Can you work these out from the model? Positions are in its coordinate system, mm. A direction names the side the tool comes from. Give positions to 0.01 mm unless a question says otherwise; leave off trailing zeros. Order: outer loops, then holes, each group sorted by start corner. A loop starts at its lowest first (then second) coordinate and runs counter-clockwise, first axis right, second up. Notation, with made-up numbers: (-36, -21) - (16, -21) arc R17 cw to (16, -17) - close; hole circle Ø7 at (-3.5, 31.5). An arc over 180 degrees is marked (long way). Return JSON: item names as keys, results as strings.
```python
from build123d import *

# Parameters (mm, degrees)
F0_W      = 101.6
F0_H      = 101.6
F1_DEPTH  = 25.4
F3_DEPTH  = 25.401
F5_DEPTH  = 76.2
F7_DEPTH  = 25.4
F9_DEPTH  = 76.2
F11_DEPTH = 25.4
F13_DEPTH = 50.8
F15_DEPTH = 25.4


with BuildPart() as f1:
    # F0 (on Front) → F1 (new body)
    with BuildSketch(Plane.XZ):
        Rectangle(F0_W, F0_H)
    extrude(amount=F1_DEPTH)

    # F2 (on face) → F3 (cut, through all)
    with BuildSketch(Plane.XZ.offset(25.4)):
        Polygon((25.4, 50.8), (-25.4, 50.8), (25.4, -10.855978), align=None)
        Polygon((-25.4, 10.855978), (-25.4, -50.8), (25.4, -50.8), align=None)
    extrude(amount=-F3_DEPTH, mode=Mode.SUBTRACT)

    # F4 (on face) → F5 (join)
    with BuildSketch(Plane(origin=(0, 0, 0), x_dir=(-1, 0, 0), z_dir=(0, 1, 0))):
        Polygon((-25.4, 50.8), (-50.8, 50.8), (-50.8, -50.8), (-25.4, -50.8), (-25.4, -10.855978), align=None)
    extrude(amount=F5_DEPTH)

    # F6 (on face) → F7 (cut)
    with BuildSketch(Plane.YZ.offset(50.8)):
        Polygon((50.8, 50.8), (0, 50.8), (50.8, -10.855978), align=None)
        Polygon((0, 10.855978), (0, -50.8), (50.8, -50.8), align=None)
    extrude(amount=-F7_DEPTH, mode=Mode.SUBTRACT)

    # F8 (on face) → F9 (join)
    with BuildSketch(Plane(origin=(25.4, 0, 0), x_dir=(0, -1, 0), z_dir=(-1, 0, 0))):
        Polygon((-50.8, -10.855978), (-50.8, 50.8), (-76.2, 50.8), (-76.2, -50.8), (-50.8, -50.8), align=None)
    extrude(amount=F9_DEPTH)

    # F10 (on face) → F11 (cut)
    with BuildSketch(Plane(origin=(0, 76.2, 0), x_dir=(-1, 0, 0), z_dir=(0, 1, 0))):
        Polygon((25.4, 50.8), (-25.4, 50.8), (25.4, -10.855978), align=None)
        Polygon((-25.4, 10.855978), (-25.4, -50.8), (25.4, -50.8), align=None)
    extrude(amount=-F11_DEPTH, mode=Mode.SUBTRACT)

    # F12 (on face) → F13 (join)
    with BuildSketch(Plane.XZ.offset(-50.8)):
        Polygon((-25.4, -10.855978), (-25.4, 50.8), (-50.8, 50.8), (-50.8, -50.8), (-25.4, -50.8), align=None)
    extrude(amount=F13_DEPTH)

    # F14 (on face) → F15 (cut)
    with BuildSketch(Plane(origin=(-50.8, 0, 0), x_dir=(0, -1, 0), z_dir=(-1, 0, 0))):
        Polygon((0, 50.8), (-50.8, 50.8), (0, -10.855978), align=None)
        Polygon((-50.8, 10.855978), (-50.8, -50.8), (0, -50.8), align=None)
    extrude(amount=-F15_DEPTH, mode=Mode.SUBTRACT)


solid = f1.part
```
1. On a 3-axis mill with a long thin cutter (end or side, diameter ignored), from which of +Z, -Z, +X, -X, +Y, -Y can I reach the whole of each face in a straight line? I mean faces 1 (the face through (-25.4, 26, -1)), 2 (the face through (38.278, 25.756, -20.404)), 3 (the face through (-0.356, 63.678, -20.404)), 4 (the face through (0.356, -12.878, -20.404)), 5 (the face through (38.278, 25.044, 20.404)). Say none if no direction works.
Checks:
{"face 1": "none", "face 2": "-Z, +X", "face 3": "-Z, +Y", "face 4": "-Z, -Y", "face 5": "+Z, +X"}
2. Suppose I cut it at A-A (z = -34.5). List the corners of the cut face in (x, y) for me.
Checks:
{"outline": "(-50.8, -25.4) - (-25.4, -25.4) - (-25.4, 13.43) - (-50.8, 13.43) - close; (-50.8, 50.8) - (-11.97, 50.8) - (-11.97, 76.2) - (-50.8, 76.2) - close; (11.97, -25.4) - (50.8, -25.4) - (50.8, 0) - (11.97, 0) - close; (25.4, 37.37) - (50.8, 37.37) - (50.8, 76.2) - (25.4, 76.2) - close"}
3. If I drill on L1, parallel to Y at x = 31, z = -1.5; L2, parallel to X at y = 32.5, z = 3.5; L3, parallel to Y at x = 33, z = -7, over which ranges is the centre line in solid material (lowest first)? Write a range as [from, to].
Checks:
{"L1": "[-25.4, 0], [10.18, 43.09], [50.8, 76.2]", "L2": "[-50.8, -25.4], [25.4, 50.8]", "L3": "[-25.4, 0], [14.71, 47.62], [50.8, 76.2]"}
4. Suppose I cut it at C-C (x = -4.5). List the corners of the cut face in (y, z) for me.
Checks:
{"outline": "(-25.4, -14.51) - (0, -14.51) - (0, 25.43) - (-25.4, 25.43) - close; (50.8, -25.43) - (76.2, -25.43) - (76.2, 14.51) - (50.8, 14.51) - close"}
5. For pin 1 Ø1 at (x, z) = (-22.5, 38.5) entering from +Y; pin 2 Ø5 at (x, y) = (11, 64.5) entering from -Z, each with a flat end and sliding along its axis, tell me the tip position at first contact or that it passes through.
Checks:
{"pin 1": "y = 0", "pin 2": "z = -9.66"}
6. Suppose I cut it at B-B (y = -10). List the corners of the cut face in (x, z) for me.
Checks:
{"outline": "(-50.8, -50.8) - (-25.4, -50.8) - (-25.4, 10.86) - (25.4, -50.8) - (50.8, -50.8) - (50.8, 50.8) - (25.4, 50.8) - (25.4, -10.86) - (-25.4, 50.8) - (-50.8, 50.8) - close"}
7. Suppose I cut it at D-D (y = 16). List the corners of the cut face in (x, z) for me, plus the area to 3 significant figures.
Checks:
{"outline": "(-50.8, -31.38) - (-25.4, -31.38) - (-25.4, 8.56) - (-50.8, 8.56) - close; (25.4, -8.56) - (50.8, -8.56) - (50.8, 31.38) - (25.4, 31.38) - close", "area": "2,030 mm^2"}
8. Thinking about a two-plate mould opening in Y: for faces 6 (the face through (-1, 50.8, 1)), 7 (the face through (-38.278, 25.044, -20.404)), 8 (the face through (38, -13, -50.8)), 9 (the face through (-1, -25.4, 1)), which applies, +Y half, -Y half, draft (parallel to the pull), parting line (faces both ways), or undercut?
Checks:
{"face 6": "undercut", "face 7": "undercut", "face 8": "draft", "face 9": "-Y half"}
